from build123d import *

# Parameters (mm, degrees)
F1_DEPTH = 12.7
F2_W     = 12.7
F2_H     = 59.960696
F3_DEPTH = 38.1
F5_DEPTH = 25.4
F7_DEPTH = 25.4
F8_R     = 5.786168
F8_R_2   = 6.967472
F9_DEPTH = 25.4


with BuildPart() as f1:
    # F0 (on Right) → F1 (new body)
    with BuildSketch(Plane.YZ):
        Polygon((-109.703772, 19.6246), (-82.661435, -27.145265), (87.22869, -27.145265), (87.22869, 125.254735), (25.250674, 115.436092), (-28.360057, 9.155148), (-79.160057, 9.155148), (-99.851914, 23.26324), align=None)
    extrude(amount=F1_DEPTH)

    # F2 (on face) → F3 (join)
    with BuildSketch(Plane(origin=(0, 0, -27.145265), x_dir=(1, 0, 0), z_dir=(0, 0, -1))):
        with Locations((6.35, -57.248342)):
            Rectangle(F2_W, F2_H)
    extrude(amount=F3_DEPTH)

    # F4 (on face) → F5 (cut)
    with BuildSketch(Plane.YZ.offset(12.7)):
        Polygon((73.597223, -65.245265), (27.267994, -27.145265), (27.267994, -65.245265), align=None)
    extrude(amount=-F5_DEPTH, mode=Mode.SUBTRACT)

    # F6 (on face) → F7 (join)
    with BuildSketch(Plane(origin=(0, 0, 0), x_dir=(0, -1, 0), z_dir=(-1, 0, 0))):
        Polygon((-87.22869, 125.254735), (-87.22869, -65.245265), (-73.597223, -65.245265), (-73.597223, 123.095219), align=None)
    extrude(amount=F7_DEPTH)

    # F8 (on face) → F9 (cut)
    with BuildSketch(Plane.XZ.offset(-73.597223)):
        with Locations((-13.092614, 110.243045)):
            Circle(F8_R)
        with Locations((-12.68347, -48.504848)):
            Circle(F8_R_2)
    extrude(amount=-F9_DEPTH, mode=Mode.SUBTRACT)


solid = f1.part
Source: CAD feature listing. Evaluate the final solid. Frame: model axes, mm. A direction names the side the tool comes from. Give positions to 0.01 mm unless a question says otherwise; leave off trailing zeros. Write each loop counter-clockwise with the first axis right and the second up, starting at its lowest first coordinate (ties: lowest second). Pieces come first, ordered by that corner, then holes. Notation, with made-up numbers: (13, 49) -> (56, 49) arc R10 ccw to (56, 66) -> close; hole circle Ø6 at (22.25, -31.5). An arc over 180 degrees is marked (long way). Write item = value, one per line.
Q1. Mould query, pull axis Z, two halves, no side actions, for faces 1 (the face through (-6, 81, -65.245)), 2 (the face through (-18.213, 80.318, -52.744)), 3 (the face through (-14.347, 80.318, 104.594)), 4 (the face through (6.26, -104.71, 21.47)). Classes: +Z half, -Z half, draft (parallel to the pull), parting line (faces both ways), or undercut.
Here are the results:
face_1 = -Z half
face_2 = undercut
face_3 = undercut
face_4 = +Z half
Q2. Reachability of faces 5 (the face through (6, -28, -27.145)), 6 (the face through (-25.4, 81, 31)), 7 (the face through (0, 24, 30)), 8 (the face through (6.26, -89.36, 16.11)), 9 (the face through (12.7, 34, 31)) from +Z, -Z, +X, -X, +Y, -Y: full face, straight path, thin tool, end or side. Return the list, or none.
Here are the results:
face_5 = -Z, +X, -X, -Y
face_6 = +Z, -Z, -X, +Y, -Y
face_7 = +Z, -Z, -X, -Y
face_8 = +Z, +X, -X
face_9 = +Z, -Z, +X, +Y, -Y
Q3. First-contact query: pin 1 (9.5 mm diameter, centred on x = -13.09, z = 110.24, fed in from -Y); pin 2 (6.5 mm diameter, centred on x = 3.5, y = -47.5, fed in from +Z); pin 3 (14 mm diameter, centred on x = 4, y = -47.5, fed in from -Z); pin 4 (20.5 mm diameter, centred on x = -17.5, z = 37, fed in from -Y). Flat tips, straight axial feed; report the tip coordinate or a pass-through.
Here are the results:
pin_1 = through
pin_2 = 9.16
pin_3 = -27.15
pin_4 = 73.6
Q4. Line query: line 1 (Z direction, x = -15, y = 76.5); line 2 (Y direction, x = -20.5, z = -55); line 3 (X direction, y = 54, z = 7). Output: solid intervals per line, ascending. Write a range as from..to.
Here are the results:
line_1 = -65.25..-55.08, -41.93..104.78, 115.71..123.56
line_2 = 73.6..87.23
line_3 = 0..12.7
Q5. Cut plane B-B on x = 6. Return loops of the section in (y, z), then the cut area to 3 significant figures.
Here are the results:
outline = (-109.7, 19.62) -> (-82.66, -27.15) -> (27.27, -27.15) -> (73.6, -65.25) -> (87.23, -65.25) -> (87.23, 125.25) -> (25.25, 115.44) -> (-28.36, 9.16) -> (-79.16, 9.16) -> (-99.85, 23.26) -> close
area = 17,900 mm²
Q6. Cut plane A-A on x = -13.5. Return loops of the section in (y, z).
Here are the results:
outline = (73.6, -65.25) -> (87.23, -65.25) -> (87.23, -55.42) -> (73.6, -55.42) -> close; (73.6, -41.59) -> (87.23, -41.59) -> (87.23, 104.47) -> (73.6, 104.47) -> close; (73.6, 116.01) -> (87.23, 116.01) -> (87.23, 125.25) -> (73.6, 123.1) -> close
Q7. Cut plane C-C on y = -62. Return loops of the section in (x, z), then the cut area to 3 significant figures.
Here are the results:
outline = (0, -27.15) -> (12.7, -27.15) -> (12.7, 9.16) -> (0, 9.16) -> close
area = 461 mm²
Q8. Cut plane D-D on z = -37.5. Return loops of the section in (x, y), then the cut area to 3 significant figures.
Here are the results:
outline = (-25.4, 73.6) -> (0, 73.6) -> (0, 39.86) -> (12.7, 39.86) -> (12.7, 87.23) -> (-25.4, 87.23) -> close
area = 948 mm²
